from build123d import *

# Parameters (mm, degrees)
SKETCH1_W                      = 240
SKETCH1_H                      = 133.2
BOSS_EXTRUDE1_DEPTH            = 13
SKETCH32_W                     = 20
SKETCH32_H                     = 133.2
CUT_EXTRUDE10_DEPTH            = 10
FILLET1_START                  = -68
FILLET1_DEPTH                  = 136
FILLET1_START_2                = -66.6
FILLET1_2_DEPTH                = 133.2
M6X1_0_TAPPED_HOLE1_D          = 5
M6X1_0_TAPPED_HOLE1_DEPTH      = 15
M6X1_0_TAPPED_HOLE1_TIP        = 1.502151548
SKETCH36_W                     = 96
SKETCH36_H                     = 35
CUT_EXTRUDE11_DEPTH            = 7
SKETCH37_W                     = 76
SKETCH37_H                     = 35
CUT_EXTRUDE12_DEPTH            = 144.991527529
M4X0_7_TAPPED_HOLE1_AT_2_COUNT = 2
M4X0_7_TAPPED_HOLE1_AT_2_PITCH = 20
M4X0_7_TAPPED_HOLE1_AT_3_COUNT = 2
M4X0_7_TAPPED_HOLE1_AT_3_PITCH = 86
M4X0_7_TAPPED_HOLE1_AT_4_COUNT = 2
M4X0_7_TAPPED_HOLE1_AT_4_PITCH = 88.294960219
LPATTERN1_COUNT                = 3
LPATTERN1_PITCH                = 41
LPATTERN1_COUNT_DIR2           = 2
LPATTERN1_PITCH_DIR2           = 104
CHAMFER1_SIZE                  = 3


with BuildPart() as part:
    # Sketch1 → Boss-Extrude1 (new body)
    with BuildSketch(Plane(origin=(0, 0, 0), x_dir=(1, 0, 0), z_dir=(0, 1, 0))):
        with Locations((7, 0)):
            Rectangle(SKETCH1_W, SKETCH1_H)
    extrude(amount=BOSS_EXTRUDE1_DEPTH)

    # Sketch32 → Cut-Extrude10 (cut)
    with BuildSketch(Plane.XZ):
        with Locations((117, 0)):
            Rectangle(SKETCH32_W, SKETCH32_H)
    extrude(amount=-CUT_EXTRUDE10_DEPTH, mode=Mode.SUBTRACT)

    # Fillet1: read off the stored shape, not the designer's step
    # Fillet1 outline → Fillet1 (cut)
    with BuildSketch(Plane.XY.offset(FILLET1_START)):
        with BuildLine():
            Line((107, 0), (107, 5))
            ThreePointArc((107, 5), (105.535533906, 1.464466094), (102, 0))
            Line((102, 0), (107, 0))
        make_face()
    extrude(amount=FILLET1_DEPTH, mode=Mode.SUBTRACT)

    # Fillet1 2 outline → Fillet1 2 (add)
    with BuildSketch(Plane.XY.offset(FILLET1_START_2)):
        with BuildLine():
            ThreePointArc((107, 5), (108.464466094, 8.535533906), (112, 10))
            Line((112, 10), (107, 10))
            Line((107, 10), (107, 5))
        make_face()
    extrude(amount=FILLET1_2_DEPTH)

    # M6x1.0 Tapped Hole1
    with Locations(Plane(origin=(0, 13, 0), x_dir=(1, 0, 0), z_dir=(0, 1, 0))):
        with Locations((119.05, 60.25), (119.05, 15.75), (119.05, -16.05), (119.05, -60.55)):
            Hole(M6X1_0_TAPPED_HOLE1_D / 2, depth=M6X1_0_TAPPED_HOLE1_DEPTH)
            with Locations((0, 0, -(M6X1_0_TAPPED_HOLE1_DEPTH + M6X1_0_TAPPED_HOLE1_TIP / 2))):  # 118° drill point
                Cone(0, M6X1_0_TAPPED_HOLE1_D / 2, M6X1_0_TAPPED_HOLE1_TIP, mode=Mode.SUBTRACT)

    # Sketch36 → Cut-Extrude11 (cut)
    with BuildSketch(Plane(origin=(0, 13, 0), x_dir=(1, 0, 0), z_dir=(0, 1, 0))):
        with Locations((-57, -41.1)):
            Rectangle(SKETCH36_W, SKETCH36_H)
        with Locations((-57, -0.1)):
            Rectangle(SKETCH36_W, SKETCH36_H)
        with Locations((-57, 40.9)):
            Rectangle(SKETCH36_W, SKETCH36_H)
        with Locations((47, 40.9)):
            Rectangle(SKETCH36_W, SKETCH36_H)
        with Locations((47, -0.1)):
            Rectangle(SKETCH36_W, SKETCH36_H)
        with Locations((47, -41.1)):
            Rectangle(SKETCH36_W, SKETCH36_H)
    extrude(amount=-CUT_EXTRUDE11_DEPTH, mode=Mode.SUBTRACT)

    # Sketch37 → Cut-Extrude12 (cut, through all)
    with BuildSketch(Plane(origin=(0, 13, 0), x_dir=(1, 0, 0), z_dir=(0, 1, 0))):
        with Locations((-57, -41.1)):
            Rectangle(SKETCH37_W, SKETCH37_H)
        with Locations((-57, -0.1)):
            Rectangle(SKETCH37_W, SKETCH37_H)
        with Locations((-57, 40.9)):
            Rectangle(SKETCH37_W, SKETCH37_H)
        with Locations((47, -0.1)):
            Rectangle(SKETCH37_W, SKETCH37_H)
        with Locations((47, -41.1)):
            Rectangle(SKETCH37_W, SKETCH37_H)
        with Locations((47, 40.9)):
            Rectangle(SKETCH37_W, SKETCH37_H)
    extrude(amount=-CUT_EXTRUDE12_DEPTH, mode=Mode.SUBTRACT)

    # Sketch39 → M4x0.7 Tapped Hole1 (revolve, cut)
    with BuildSketch(Plane(origin=(-100, 6, 51.1), x_dir=(0, 0, 1), z_dir=(1, 0, 0))):
        Polygon((0, 0), (0, 11.091420021), (1.65, 10.1), (1.65, 0), align=None)
    m4x0_7_tapped_hole1 = revolve(axis=Axis((-100, 12.35, 51.1), (0, -1, 0)), mode=Mode.SUBTRACT)

    # M4x0.7 Tapped Hole1 at 2: M4x0.7 Tapped Hole1 ×2
    with Locations(*[(0, 0, -i * M4X0_7_TAPPED_HOLE1_AT_2_PITCH) for i in range(1, M4X0_7_TAPPED_HOLE1_AT_2_COUNT)]):
        add(m4x0_7_tapped_hole1, mode=Mode.SUBTRACT)

    # M4x0.7 Tapped Hole1 at 3: M4x0.7 Tapped Hole1 ×2
    with Locations(*[(i * M4X0_7_TAPPED_HOLE1_AT_3_PITCH, 0, 0) for i in range(1, M4X0_7_TAPPED_HOLE1_AT_3_COUNT)]):
        add(m4x0_7_tapped_hole1, mode=Mode.SUBTRACT)

    # M4x0.7 Tapped Hole1 at 4: M4x0.7 Tapped Hole1 ×2
    with Locations(*[Vector(0.9740080270391964, 0, -0.22651349466027837) * (i * M4X0_7_TAPPED_HOLE1_AT_4_PITCH) for i in range(1, M4X0_7_TAPPED_HOLE1_AT_4_COUNT)]):
        add(m4x0_7_tapped_hole1, mode=Mode.SUBTRACT)

    # LPattern1: M4x0.7 Tapped Hole1 3 × 2
    with Locations(*[(j * LPATTERN1_PITCH_DIR2, 0, -i * LPATTERN1_PITCH) for i in range(LPATTERN1_COUNT) for j in range(LPATTERN1_COUNT_DIR2) if (i, j) != (0, 0)]):
        add(m4x0_7_tapped_hole1, mode=Mode.SUBTRACT)

    # LPattern1 copy 1 sketch → LPattern1 copy 1 (revolve, cut)
    with BuildSketch(Plane(origin=(4, 6, 31.1), x_dir=(0, 0, 1), z_dir=(1, 0, 0))):
        Polygon((0, 0), (0, 11.091420021), (1.65, 10.1), (1.65, 0), align=None)
    revolve(axis=Axis((4, 12.35, 31.1), (0, -1, 0)), mode=Mode.SUBTRACT)

    # LPattern1 copy 2 sketch → LPattern1 copy 2 (revolve, cut)
    with BuildSketch(Plane(origin=(-100, 6, -9.9), x_dir=(0, 0, 1), z_dir=(1, 0, 0))):
        Polygon((0, 0), (0, 11.091420021), (1.65, 10.1), (1.65, 0), align=None)
    revolve(axis=Axis((-100, 12.35, -9.9), (0, -1, 0)), mode=Mode.SUBTRACT)

    # LPattern1 copy 3 sketch → LPattern1 copy 3 (revolve, cut)
    with BuildSketch(Plane(origin=(4, 6, -9.9), x_dir=(0, 0, 1), z_dir=(1, 0, 0))):
        Polygon((0, 0), (0, 11.091420021), (1.65, 10.1), (1.65, 0), align=None)
    revolve(axis=Axis((4, 12.35, -9.9), (0, -1, 0)), mode=Mode.SUBTRACT)

    # LPattern1 copy 4 sketch → LPattern1 copy 4 (revolve, cut)
    with BuildSketch(Plane(origin=(-100, 6, -50.9), x_dir=(0, 0, 1), z_dir=(1, 0, 0))):
        Polygon((0, 0), (0, 11.091420021), (1.65, 10.1), (1.65, 0), align=None)
    revolve(axis=Axis((-100, 12.35, -50.9), (0, -1, 0)), mode=Mode.SUBTRACT)

    # LPattern1 copy 5 sketch → LPattern1 copy 5 (revolve, cut)
    with BuildSketch(Plane(origin=(4, 6, -50.9), x_dir=(0, 0, 1), z_dir=(1, 0, 0))):
        Polygon((0, 0), (0, 11.091420021), (1.65, 10.1), (1.65, 0), align=None)
    revolve(axis=Axis((4, 12.35, -50.9), (0, -1, 0)), mode=Mode.SUBTRACT)

    # LPattern1 copy 6 sketch → LPattern1 copy 6 (revolve, cut)
    with BuildSketch(Plane(origin=(90, 6, 51.1), x_dir=(0, 0, 1), z_dir=(1, 0, 0))):
        Polygon((0, 0), (0, 11.091420021), (1.65, 10.1), (1.65, 0), align=None)
    revolve(axis=Axis((90, 12.35, 51.1), (0, -1, 0)), mode=Mode.SUBTRACT)

    # LPattern1 copy 7 sketch → LPattern1 copy 7 (revolve, cut)
    with BuildSketch(Plane(origin=(-14, 6, 10.1), x_dir=(0, 0, 1), z_dir=(1, 0, 0))):
        Polygon((0, 0), (0, 11.091420021), (1.65, 10.1), (1.65, 0), align=None)
    revolve(axis=Axis((-14, 12.35, 10.1), (0, -1, 0)), mode=Mode.SUBTRACT)

    # LPattern1 copy 8 sketch → LPattern1 copy 8 (revolve, cut)
    with BuildSketch(Plane(origin=(90, 6, 10.1), x_dir=(0, 0, 1), z_dir=(1, 0, 0))):
        Polygon((0, 0), (0, 11.091420021), (1.65, 10.1), (1.65, 0), align=None)
    revolve(axis=Axis((90, 12.35, 10.1), (0, -1, 0)), mode=Mode.SUBTRACT)

    # LPattern1 copy 9 sketch → LPattern1 copy 9 (revolve, cut)
    with BuildSketch(Plane(origin=(-14, 6, -30.9), x_dir=(0, 0, 1), z_dir=(1, 0, 0))):
        Polygon((0, 0), (0, 11.091420021), (1.65, 10.1), (1.65, 0), align=None)
    revolve(axis=Axis((-14, 12.35, -30.9), (0, -1, 0)), mode=Mode.SUBTRACT)

    # LPattern1 copy 10 sketch → LPattern1 copy 10 (revolve, cut)
    with BuildSketch(Plane(origin=(90, 6, -30.9), x_dir=(0, 0, 1), z_dir=(1, 0, 0))):
        Polygon((0, 0), (0, 11.091420021), (1.65, 10.1), (1.65, 0), align=None)
    revolve(axis=Axis((90, 12.35, -30.9), (0, -1, 0)), mode=Mode.SUBTRACT)

    # LPattern1 copy 11 sketch → LPattern1 copy 11 (revolve, cut)
    with BuildSketch(Plane(origin=(90, 6, 31.1), x_dir=(0, 0, 1), z_dir=(1, 0, 0))):
        Polygon((0, 0), (0, 11.091420021), (1.65, 10.1), (1.65, 0), align=None)
    revolve(axis=Axis((90, 12.35, 31.1), (0, -1, 0)), mode=Mode.SUBTRACT)

    # LPattern1 copy 12 sketch → LPattern1 copy 12 (revolve, cut)
    with BuildSketch(Plane(origin=(-14, 6, -9.9), x_dir=(0, 0, 1), z_dir=(1, 0, 0))):
        Polygon((0, 0), (0, 11.091420021), (1.65, 10.1), (1.65, 0), align=None)
    revolve(axis=Axis((-14, 12.35, -9.9), (0, -1, 0)), mode=Mode.SUBTRACT)

    # LPattern1 copy 13 sketch → LPattern1 copy 13 (revolve, cut)
    with BuildSketch(Plane(origin=(90, 6, -9.9), x_dir=(0, 0, 1), z_dir=(1, 0, 0))):
        Polygon((0, 0), (0, 11.091420021), (1.65, 10.1), (1.65, 0), align=None)
    revolve(axis=Axis((90, 12.35, -9.9), (0, -1, 0)), mode=Mode.SUBTRACT)

    # LPattern1 copy 14 sketch → LPattern1 copy 14 (revolve, cut)
    with BuildSketch(Plane(origin=(-14, 6, -50.9), x_dir=(0, 0, 1), z_dir=(1, 0, 0))):
        Polygon((0, 0), (0, 11.091420021), (1.65, 10.1), (1.65, 0), align=None)
    revolve(axis=Axis((-14, 12.35, -50.9), (0, -1, 0)), mode=Mode.SUBTRACT)

    # LPattern1 copy 15 sketch → LPattern1 copy 15 (revolve, cut)
    with BuildSketch(Plane(origin=(90, 6, -50.9), x_dir=(0, 0, 1), z_dir=(1, 0, 0))):
        Polygon((0, 0), (0, 11.091420021), (1.65, 10.1), (1.65, 0), align=None)
    revolve(axis=Axis((90, 12.35, -50.9), (0, -1, 0)), mode=Mode.SUBTRACT)

    # Chamfer1
    chamfer1_edges = [part.edges().sort_by_distance(p)[0] for p in [
        (-95, 6, -40.9),
        (-19, 6, -40.9),
        (-95, 6, 0.1),
        (-19, 6, 0.1),
        (-19, 6, 41.1),
        (-95, 6, 41.1),
        (9, 6, -40.9),
        (85, 6, -40.9),
        (85, 6, 0.1),
        (9, 6, 0.1),
        (9, 6, 41.1),
        (85, 6, 41.1),
        (7, 13, -66.6),
        (127, 13, 0),
        (7, 13, 66.6),
    ]]
    chamfer(chamfer1_edges, length=CHAMFER1_SIZE - 0.0001)  # a hair under: the kernel refuses the full size


solid = part.part
Model file for the job. Use its own axes, mm. A direction names the side the tool comes from. Give positions to 0.01 mm unless a question says otherwise; leave off trailing zeros. Loops run counter-clockwise (first coordinate to the right, second up) from the corner with the lowest first, then second, coordinate; pieces in that order, holes last. Notation, with made-up numbers: (4.5, 3) - (34.5, 3) arc R31 ccw to (34.5, 34) - close; hole circle Ø3 at (-11, 72). An arc over 180 degrees is marked (long way). Use one line per item in the form item = value.
(1) 3-axis set-ups, long thin cutter, end or side, ignore diameter. For faces 4 (the face through (116.665, 11.479, -16.501)), 5 (the face through (46, 7, 23.6)): which of +Z, -Z, +X, -X, +Y, -Y reach the whole face in a straight line?
Determined:
face_4 = +Y, -Y
face_5 = +Y
(2) Drop flat-ended pins along their axis: P1, Ø1, axis at y = 5.5, z = -13, coming from the +X side; P2, Ø4, axis at x = 5, z = -26.5, coming from the +Y side; P3, Ø3, axis at x = 90, z = -50.9, coming from the -Y side; P4, Ø0.9, axis at y = 2, z = -1.5, coming from the +X side. Give the stop position or say it passes through.
Determined:
P1 = 107.1
P2 = 6
P3 = through
P4 = 106.3
(3) Cut at A-A (z = -41). Count the separate pieces of the cut face and the enclosed holes in it, then the cut area to 4 significant figures.
Determined:
separate_pieces = 3
enclosed_holes = 0
area = 641.5 mm^2
(4) Cut at B-B (x = -70). Give the cut face in (y, z), then the cut area to 3 significant figures.
Determined:
outline = (0, -66.6) - (10, -66.6) - (13, -63.6) - (13, -58.4) - (0, -58.4) - close; (0, -23.4) - (13, -23.4) - (13, -17.4) - (0, -17.4) - close; (0, 17.6) - (13, 17.6) - (13, 23.6) - (0, 23.6) - close; (0, 58.6) - (13, 58.6) - (13, 63.6) - (10, 66.6) - (0, 66.6) - close
area = 358 mm^2
(5) Pull direction Z, two halves, no side cores. Call faces 1 (the face through (-7, 0, -16)), 2 (the face through (-58, 7, -17.4)), 3 (the face through (-21, 5, 66.6)): pulls with the +Z half, pulls with the -Z half, needs draft (parallel to the pull), parting line crosses it, or undercut.
Determined:
face_1 = needs draft
face_2 = undercut
face_3 = pulls with the +Z half
(6) Drill centre lines: L1, parallel to Z at x = 41.5, y = 4.75; L2, parallel to X at y = 2.5, z = 17; L3, parallel to X at y = 7, z = -43. Where is each one in solid material? Low to high.
Determined:
L1 = -66.6 to -58.4, -23.4 to -17.4, 17.6 to 23.6, 58.6 to 66.6
L2 = -113 to -95, -19 to 9, 85 to 106.33
L3 = -113 to -105, -9 to -1, 95 to 107.42
